```python
from build123d import *

# Parameters (mm, degrees)
F0_W = 238.76
F0_H = 81.28
F2_T = -30.48
F3_R = 12.7


with BuildPart() as f1:
    # F0 (on Front) → F1 (revolve)
    with BuildSketch(Plane.XZ):
        with Locations((-119.38, 40.64)):
            Rectangle(F0_W, F0_H)
    revolve(axis=Axis((0, 0, 40.64), (0, 0, -1)))

    # F2
    f2_openings = [f1.faces().sort_by_distance(p)[0] for p in [
        (0, 0, 0),
    ]]
    offset(amount=F2_T, openings=f2_openings)

    # F3
    f3_edges = [f1.edges().sort_by_distance(p)[0] for p in [
        (238.76, 0, 81.28),
        (238.76, 0, 0),
        (208.28, 0, 0),
    ]]
    fillet(f3_edges, radius=F3_R)


solid = f1.part
```
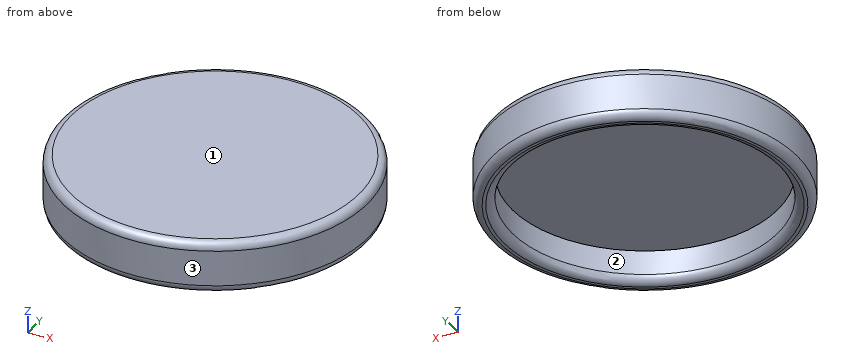
The model under review builds one solid part; all positions refer to its coordinate system, in mm. Face numbers are marked on the shaded views. Round coordinates to 2 decimals unless told otherwise and drop trailing zeros. Order: outer loops, then holes, each group sorted by start corner. A loop starts at its lowest first (then second) coordinate and runs counter-clockwise, first axis right, second up. Notation, with made-up numbers: (-27, 55.5) -> (9, 55.5) arc R13 ccw to (9, 69.5) -> close; hole circle Ø11 at (30, -35). An arc over 180 degrees is marked (long way). Use a Markdown table: item, result.
Q1. We need section A-A on x = 0. Write out the cut boundary in (y, z), then the cut area to 3 significant figures.
Values:
| item | result |
|---|---|
| outline | (-238.76, 12.7) arc R12.7 ccw to (-226.06, 0) -> (-220.98, 0) arc R12.7 ccw to (-208.28, 12.7) -> (-208.28, 50.8) -> (208.28, 50.8) -> (208.28, 12.7) arc R12.7 ccw to (220.98, 0) -> (226.06, 0) arc R12.7 ccw to (238.76, 12.7) -> (238.76, 68.58) arc R12.7 ccw to (226.06, 81.28) -> (-226.06, 81.28) arc R12.7 ccw to (-238.76, 68.58) -> close |
| area | 17,400 mm^2 |
Q2. Mouldability with a two-part tool opening along Y and no side actions: class the marked faces 1, 2 and 3 as +Y half, -Y half, draft (parallel to the pull), parting line (faces both ways), or undercut.
Values:
| item | result |
|---|---|
| face 1 | draft |
| face 2 | undercut |
| face 3 | parting line |
Q3. Clearance check with flat-ended pins moving along their axes: P1, Ø1.5, axis at x = 48, z = 53, coming from the +Y side; P2, Ø10, axis at x = -170.5, z = 11.5, coming from the -Y side; P3, Ø5, axis at x = -84, y = 2.5, coming from the -Z side. State where each tip first meets the part, or that it passes through.
Values:
| item | result |
|---|---|
| P1 | stops at y = 234.04 |
| P2 | stops at y = -172.04 |
| P3 | stops at z = 50.8 |
Q4. We need section B-B on z = 34.5. Write out the cut boundary in (x, y), then the cut area to 3 significant figures.
Values:
| item | result |
|---|---|
| outline | circle Ø477.52 at (0, 0); hole circle Ø416.56 at (0, 0) |
| area | 42,800 mm^2 |
Q5. For line 1 (Y direction, x = 0, z = 38); line 2 (Z direction, x = -80, y = 165); line 3 (Y direction, x = -180, z = 50), list the stretches that pass through material, from the lowest coordinate up.
Values:
| item | result |
|---|---|
| line 1 | y = -238.76 to -208.28, 208.28 to 238.76 |
| line 2 | z = 50.8 to 81.28 |
| line 3 | y = -156.86 to -104.79, 104.79 to 156.86 |
